Part model, mm, in its own coordinate system. A direction names the side the tool comes from. Give positions to 0.01 mm unless a question says otherwise; leave off trailing zeros. Order: outer loops, then holes, each group sorted by start corner. A loop starts at its lowest first (then second) coordinate and runs counter-clockwise, first axis right, second up.
1. Slice it at A-A on y = 55. List the corners of the cut face in (x, z).
2. Which spindle directions (+Z, -Z, +X, -X, +Y, -Y) get a long thin tool onto all of the face, cutting with end or side? Do faces 5 (the flat face through (-13, 220, 48)), 6 (the flat face through (-150, 114, 1)). Say none if no direction does.
3. Probe line 1 (Z direction, x = 15.5, y = 130); line 2 (X direction, y = 20.5, z = -39.5); line 3 (Y direction, x = -124, z = -25). List the from-to ranges inside material, lowest first.
4. Slice it at B-B on x = -100. List the corners of the cut face in (y, z).
5. Slice it at C-C on z = 9. List the corners of the cut face in (x, y).
6. Drop a flat-ended pin along its axis: pin 1 Ø5 at (x, z) = (75, -23.5) entering from +Y. Give the stop position or say it passes through.
7. Mould opens along Z. For faces 1 (the flat face through (-2, 0, -1)), 2 (the flat face through (-2, 108, -65)), 3 (the flat face through (-2, 114, -45)), 4 (the flat face through (150, 114, 1)) say: +Z half, -Z half, draft (parallel to the pull), parting line (faces both ways), or undercut.
from build123d import *

# Parameters (mm, degrees)
SKETCH1_W           = 340
SKETCH1_H           = 130
SKETCH1_W_2         = 300
SKETCH1_H_2         = 90
BOSS_EXTRUDE1_DEPTH = 220
SKETCH1_2_W         = 340
SKETCH1_2_H         = 130
SKETCH1_2_W_2       = 300
SKETCH1_2_H_2       = 90
BOSS_EXTRUDE2_DEPTH = 220
BOSS_EXTRUDE3_REACH = 412.152
SKETCH2_W           = 130
SKETCH2_H           = 11.669014553


with BuildPart() as part:
    # Sketch1 → Boss-Extrude1 (new body)
    with BuildSketch(Plane(origin=(0, 0, 0), x_dir=(1, 0, 0), z_dir=(0, 1, 0))):
        Rectangle(SKETCH1_W, SKETCH1_H)
        Rectangle(SKETCH1_W_2, SKETCH1_H_2, mode=Mode.SUBTRACT)
    extrude(amount=BOSS_EXTRUDE1_DEPTH)

    # Sketch1<2> → Boss-Extrude2 (add)
    with BuildSketch(Plane(origin=(0, 0, 0), x_dir=(1, 0, 0), z_dir=(0, 1, 0))):
        Rectangle(SKETCH1_2_W, SKETCH1_2_H)
        Rectangle(SKETCH1_2_W_2, SKETCH1_2_H_2, mode=Mode.SUBTRACT)
    extrude(amount=BOSS_EXTRUDE2_DEPTH)

    # Sketch2 → Boss-Extrude3 (add, up to next)
    with BuildSketch(Plane.ZY.offset(170), mode=Mode.PRIVATE) as boss_extrude3_sk1:
        with Locations((0, 5.834507277)):
            Rectangle(SKETCH2_W, SKETCH2_H)
    boss_extrude3_tool1 = extrude(boss_extrude3_sk1.sketch, amount=-BOSS_EXTRUDE3_REACH, mode=Mode.PRIVATE) - part.part
    add(boss_extrude3_tool1.solids().sort_by_distance((-170, 5.834507, 0))[0])


solid = part.part
Data:
1. outline: (-170, -65) - (170, -65) - (170, 65) - (-170, 65) - close; hole (-150, -45) - (150, -45) - (150, 45) - (-150, 45) - close
2. face 5: +Z, -Z, +X, -X, +Y
2. face 6: +Y
3. line 1: z = -65 to -45, 45 to 65
3. line 2: x = -170 to -150, 150 to 170
3. line 3: y = 0 to 11.67
4. outline: (0, -65) - (220, -65) - (220, -45) - (11.67, -45) - (11.67, 45) - (220, 45) - (220, 65) - (0, 65) - close
5. outline: (-170, 0) - (170, 0) - (170, 220) - (150, 220) - (150, 11.67) - (-150, 11.67) - (-150, 220) - (-170, 220) - close
6. pin 1: stops at y = 11.67
7. face 1: draft
7. face 2: -Z half
7. face 3: undercut
7. face 4: undercut
